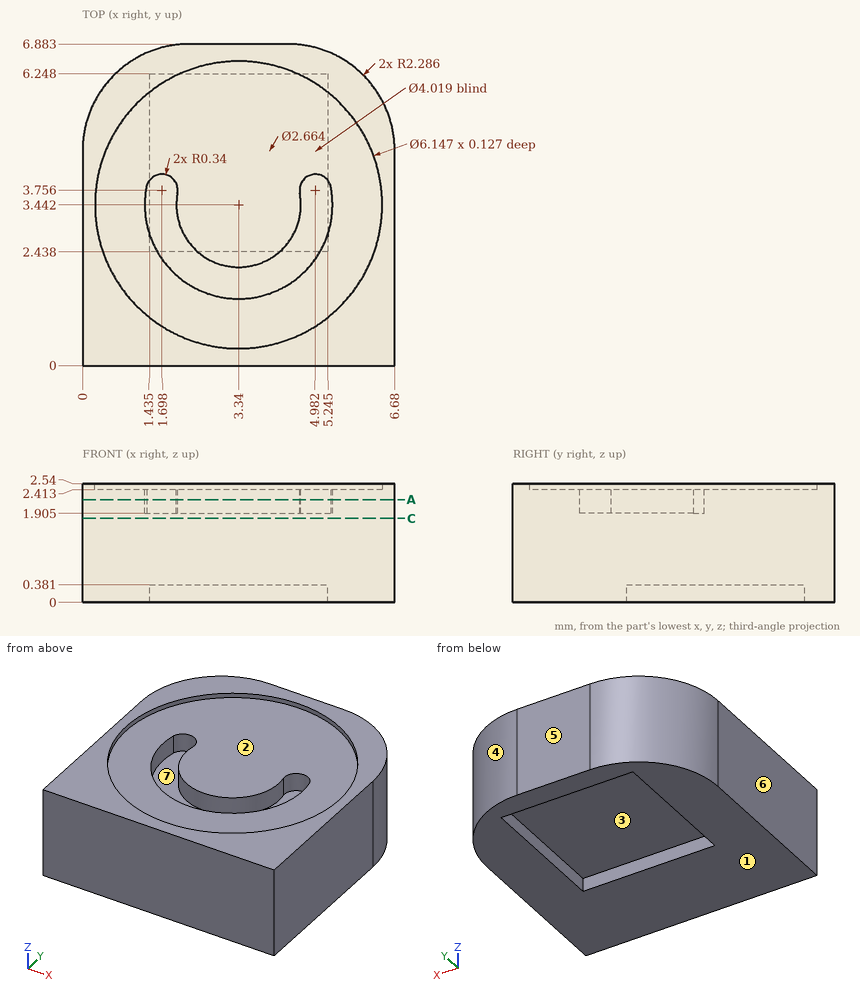
Answer from the drawing. Dimensions are ordinates in mm from the lowest x, y and z of the part. A direction names the side the tool comes from. Give positions to 0.01 mm unless a question says otherwise; leave off trailing zeros. Write each loop counter-clockwise with the first axis right and the second up, starting at its lowest first coordinate (ties: lowest second). Pieces come first, ordered by that corner, then holes. Notation, with made-up numbers: (57, 39.5) -> (93, 39.5) arc R22 ccw to (93, 56.5) -> close; hole circle Ø9 at (-5.75, 31.25). An arc over 180 degrees is marked (long way). Use a Markdown table: item, result.
(1) Section A-A, the plane z = 2.2 is taken. Determine the outline of the cut face in (x, y) (1 decimal), then the cut area to 3 significant figures.
Return value:
| item | result |
|---|---|
| outline | (0, 0) -> (6.7, 0) -> (6.7, 4.6) arc R2.3 ccw to (4.4, 6.9) -> (2.3, 6.9) arc R2.3 ccw to (0, 4.6) -> close; hole (1.4, 3.9) arc R2 ccw (long way) to (5.3, 3.9) arc R0.3 ccw to (4.6, 3.7) arc R1.3 cw (long way) to (2, 3.7) arc R0.3 ccw to start |
| area | 39.4 mm2 |
(2) Find the intervals of material crossed by probe 1 along Y at (x, z) = (3.75, 0.25); probe 2 along X at (y, z) = (3.75, 2.25) (1 decimal); probe 3 along X at (y, z) = (2.25, 2.25) (1 decimal), in increasing order. Write a range as from..to.
Return value:
| item | result |
|---|---|
| probe 1 | 0..2.44, 6.25..6.88 |
| probe 2 | 0..1.4, 2..4.6, 5.3..6.7 |
| probe 3 | 0..1.7, 2.7..3.9, 5..6.7 |
(3) For the marked faces 1, 2 and 3, determine the directions among +Z, -Z, +X, -X, +Y, -Y from which every point of the face is accessible in a straight line to the end or side of a thin tool.
Return value:
| item | result |
|---|---|
| face 1 | -Z, +X, -X, +Y, -Y |
| face 2 | +Z |
| face 3 | -Z |
(4) Flat-ended cylindrical pins translate along their axes: P1, Ø3, axis at x = 4, y = 2.5, coming from the +Z side; P2, Ø1.1, axis at x = 4, y = 3.5, coming from the -Z side; P3, Ø1.5, axis at y = 6, z = 1, coming from the -X side (1 decimal). Find the tip coordinate at first contact, or state that the pin passes through.
Return value:
| item | result |
|---|---|
| P1 | z = 2.41 |
| P2 | z = 0.38 |
| P3 | x = 0.1 |
(5) Section C-C, the plane z = 1.8 is taken. Determine the outline of the cut face in (x, y) (1 decimal).
Return value:
| item | result |
|---|---|
| outline | (0, 0) -> (6.7, 0) -> (6.7, 4.6) arc R2.3 ccw to (4.4, 6.9) -> (2.3, 6.9) arc R2.3 ccw to (0, 4.6) -> close |
(6) Determine the mould class of the marked faces 4, 5, 6 and 7 for opening direction X: released by +X, released by -X, zero draft, split by the parting line, or undercut.
Return value:
| item | result |
|---|---|
| face 4 | released by +X |
| face 5 | zero draft |
| face 6 | released by -X |
| face 7 | undercut |
